```python
from build123d import *

# Parameters (mm, degrees)
SKETCH1_R           = 50
BOSS_EXTRUDE1_DEPTH = 100
SKETCH3_R           = 15
BOSS_EXTRUDE2_DEPTH = 100
ECHELLE1_SCALE      = 0.075


with BuildPart() as part:
    # Sketch1 → Boss-Extrude1 (new body)
    with BuildSketch(Plane.XY):
        with BuildLine():
            Line((15.450849719, 47.552825815), (208.963323447, 643.122980447))
            ThreePointArc((208.963323447, 643.122980447), (210.809153806, 666.305115195), (201.968702079, 687.814761274))
            ThreePointArc((201.968702079, 687.814761274), (113.501706094, 766.442555341), (0, 800))
            ThreePointArc((0, 800), (-113.501706094, 766.442555341), (-201.968702079, 687.814761274))
            ThreePointArc((-201.968702079, 687.814761274), (-210.809153806, 666.305115195), (-208.963323447, 643.122980447))
            Line((-208.963323447, 643.122980447), (-15.450849719, 47.552825815))
            ThreePointArc((-15.450849719, 47.552825815), (0, 50), (15.450849719, 47.552825815))
        make_face()
        with Locations((0, 714.39)):
            Circle(SKETCH1_R, mode=Mode.SUBTRACT)
    extrude(amount=BOSS_EXTRUDE1_DEPTH)

    # Sketch3 → Boss-Extrude2 (add)
    with BuildSketch(Plane.XY):
        with Locations((0, 630)):
            Circle(SKETCH3_R)
    extrude(amount=-BOSS_EXTRUDE2_DEPTH)


with BuildPart() as part_1:
    # Echelle1: scaled about (0, 496.714078895, 49.597985562)
    add(part.part.scale(ECHELLE1_SCALE).moved(Location((0, 459.460522978, 45.878136645))))


solid = part_1.part
```
The listing builds one solid part. Answer for the finished solid, in the listing's coordinates (mm). A direction names the side the tool comes from. Coordinates: 2 decimals unless noted, no trailing zeros. Write each loop counter-clockwise with the first axis right and the second up, starting at its lowest first coordinate (ties: lowest second). Pieces come first, ordered by that corner, then holes. Notation, with made-up numbers: (57.25, -28.75) - (72.25, -28.75) arc R10 ccw to (72.25, -24.75) - close; hole circle Ø5 at (72, -1.5). An arc over 180 degrees is marked (long way). One line per item, written item: value.
1) Find section B-B (x = 7.5). Give the vertices of the cut face in (y, z), and give its area (3 significant figures).
Geometry check:
outline: (482.54, 45.88) - (517.47, 45.88) - (517.47, 53.38) - (482.54, 53.38) - close
area: 262 mm2
2) Each of these flat-tipped pins is pushed along its axis until it touches: pin 1 Ø1.5 at (x, z) = (1.5, 42.5) entering from +Y; pin 2 Ø8.5 at (x, y) = (0, 513.04) entering from -Z; pin 3 Ø6 at (y, z) = (471.5, 51.5) entering from +X. Where does it stop, or does it pass through?
Geometry check:
pin 1: stops at y = 507.55
pin 2: stops at z = 45.88
pin 3: stops at x = 4.89
3) A tool of negligible diameter and unlimited length cuts with its end or side. For faces 1 (the flat face through (-8.517, 485.674, 49.576)), 2 (the cylindrical face through (-0.24, 505.61, 42.18)), from which of +Z, -Z, +X, -X, +Y, -Y can it reach the whole face along a straight path? Write none if from no direction.
Geometry check:
face 1: +Z, -Z, -X, -Y
face 2: -Z
4) Consider line 1 along Z through (x, y) = (-1, 489.5); line 2 along X through (y, z) = (497, 49.25); line 3 along X through (y, z) = (467.5, 47). Determine where each line is inside the solid, lowest interval first. Write a range as from..to.
Geometry check:
line 1: z = 45.88..53.38
line 2: x = -12.2..12.2
line 3: x = -2.61..2.61
5) Find section A-A (y = 510.5). Give the vertices of the cut face in (x, z).
Geometry check:
outline: (-15.48, 45.88) - (-2.76, 45.88) - (-2.76, 53.38) - (-15.48, 53.38) - close; (2.76, 45.88) - (15.48, 45.88) - (15.48, 53.38) - (2.76, 53.38) - close
6) For a pull along Y with two mould halves and no side action, classify faces 3 (the cylindrical face through (8.622, 516.883, 49.576)), 4 (the cylindrical face through (-15.8, 509.5, 49.6)), 5 (the cylindrical face through (-0.488, 516.758, 49.576)) as pulls with the +Y half, pulls with the -Y half, needs draft (parallel to the pull), parting line crosses it, or undercut.
Geometry check:
face 3: pulls with the +Y half
face 4: parting line crosses it
face 5: undercut
7) Find section C-C (y = 478). Give the vertices of the cut face in (x, z).
Geometry check:
outline: (-6.02, 45.88) - (6.02, 45.88) - (6.02, 53.38) - (-6.02, 53.38) - close
8) Find section D-D (z = 43). Give the vertices of the cut face in (x, y) (3 decimals).
Geometry check:
outline: circle Ø2.25 at (0, 506.711)
